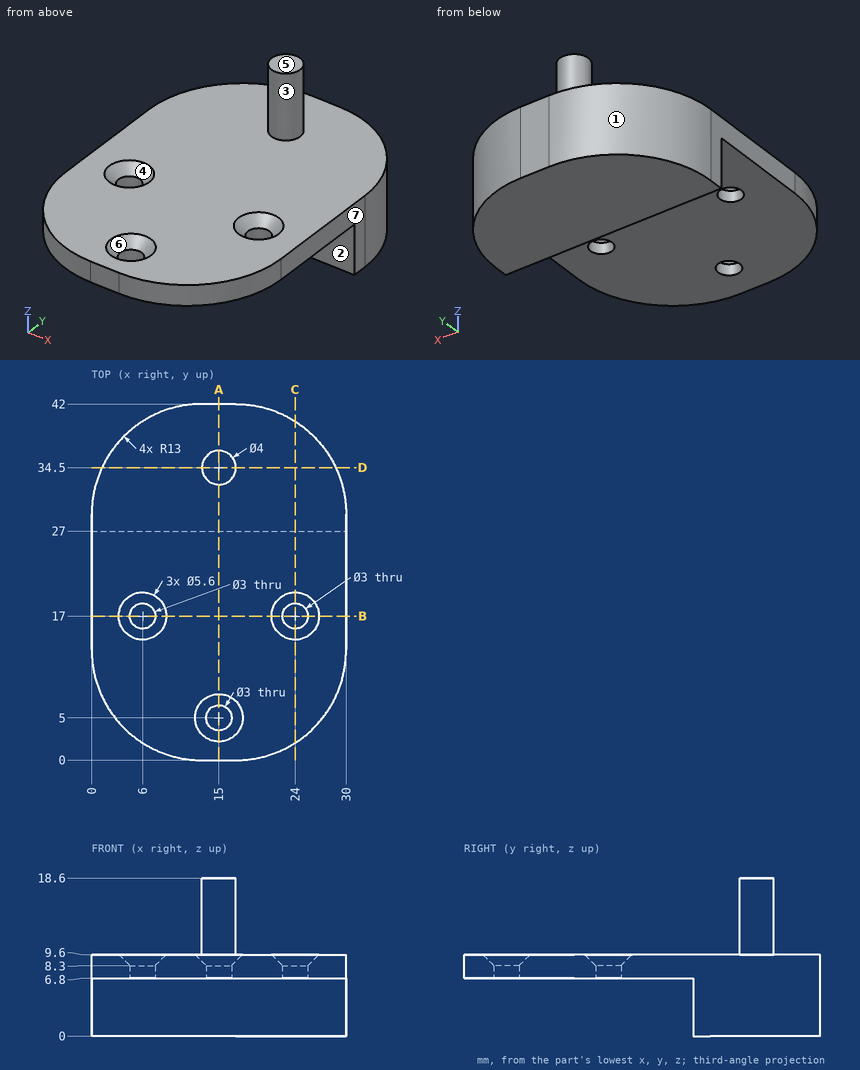
Drawing for the job (mm, zero at the part's lowest x, y, z). A direction names the side the tool comes from. Coordinates: 2 decimals unless noted, no trailing zeros. Write each loop counter-clockwise with the first axis right and the second up, starting at its lowest first coordinate (ties: lowest second). Pieces come first, ordered by that corner, then holes. Notation, with made-up numbers: (6, -0.75) -> (47, -0.75) arc R29 ccw to (47, 21.25) -> close; hole circle Ø3 at (54.5, 82). An arc over 180 degrees is marked (long way). One line per item, written item: value. Start each with the question number.
1) Slice it at B-B on y = 17. Write the cut outline in (x, z), then the cut area to 3 significant figures.
2) Slice it at A-A on x = 15. Write the cut outline in (y, z).
3) Slice it at C-C on x = 24. Write the cut outline in (y, z), then the cut area to 3 significant figures.
4) Pull direction X, two halves, no side cores. Call the marked faces 4, 5, 6 and 7: +X half, -X half, draft (parallel to the pull), parting line (faces both ways), or undercut.
5) Which spindle directions (+Z, -Z, +X, -X, +Y, -Y) get a long thin tool onto all of the face, cutting with end or side? Do the marked faces 1, 2 and 3. Say none if no direction does.
6) Flat gauge pins, fed straight in: pin 1 Ø5 at (y, z) = (36.5, 7) entering from -X; pin 2 Ø2 at (x, z) = (21, 1.5) entering from -Y; pin 3 Ø2.5 at (x, y) = (24, 17) entering from +Z; pin 4 Ø1 at (x, y) = (11.5, 12.5) entering from +Z. Where does each tip first touch, or does it go through?
7) Probe probe 1 along X at (y, z) = (17, 7.15); probe 2 along Z at (x, y) = (7, 30.5); probe 3 along Z at (x, y) = (27, 7.5). List the from-to ranges inside material, lowest first.
8) Slice it at D-D on y = 34.5. Write the cut outline in (x, z), then the cut area to 3 significant figures.
Answers follow:
1. outline: (0, 6.8) -> (4.5, 6.8) -> (4.5, 8.3) -> (3.2, 9.6) -> (0, 9.6) -> close; (7.5, 6.8) -> (22.5, 6.8) -> (22.5, 8.3) -> (21.2, 9.6) -> (8.8, 9.6) -> (7.5, 8.3) -> close; (25.5, 6.8) -> (30, 6.8) -> (30, 9.6) -> (26.8, 9.6) -> (25.5, 8.3) -> close
1. area: 63.8 mm2
2. outline: (0, 6.8) -> (3.5, 6.8) -> (3.5, 8.3) -> (2.2, 9.6) -> (0, 9.6) -> close; (6.5, 6.8) -> (27, 6.8) -> (27, 0) -> (42, 0) -> (42, 9.6) -> (36.5, 9.6) -> (36.5, 18.6) -> (32.5, 18.6) -> (32.5, 9.6) -> (7.8, 9.6) -> (6.5, 8.3) -> close
3. outline: (2.05, 6.8) -> (15.5, 6.8) -> (15.5, 8.3) -> (14.2, 9.6) -> (2.05, 9.6) -> close; (18.5, 6.8) -> (27, 6.8) -> (27, 0) -> (39.95, 0) -> (39.95, 9.6) -> (19.8, 9.6) -> (18.5, 8.3) -> close
3. area: 184 mm2
4. face 4: undercut
4. face 5: draft
4. face 6: undercut
4. face 7: +X half
5. face 1: +Z, -Z, -X, +Y
5. face 2: -Z, +X, -X, -Y
5. face 3: +Z
6. pin 1: x = 1
6. pin 2: y = 27
6. pin 3: through
6. pin 4: z = 9.6
7. probe 1: 0 to 4.5, 7.5 to 22.5, 25.5 to 30
7. probe 2: 0 to 9.6
7. probe 3: 6.8 to 9.6
8. outline: (1.22, 0) -> (28.78, 0) -> (28.78, 9.6) -> (17, 9.6) -> (17, 18.6) -> (13, 18.6) -> (13, 9.6) -> (1.22, 9.6) -> close
8. area: 301 mm2
